Input: part model. Units: mm. Frame: model coordinates. A direction names the side the tool comes from. Give positions to 0.01 mm unless a question says otherwise; leave off trailing zeros. Loops run counter-clockwise (first coordinate to the right, second up) from the corner with the lowest first, then second, coordinate; pieces in that order, holes last. Notation, with made-up numbers: M 30.25,12.5 L 49.25,12.5 A24 ccw 49.25,42.5 Z; hole C 78,21.5 d4. An arc over 180 degrees is marked long. One line per item, written item: value. Start each with the question number.
(1) Pull-direction query (Y, two-part tool) for faces 1 (the flat face through (212, 12, 320.3)), 2 (the flat face through (212, -2, 310.475)), 3 (the flat face through (212.02, -3.6, 308.96)), 4 (the flat face through (218, 0, 301)); classes: released by +Y, released by -Y, zero draft, split by the parting line, or undercut.
(2) Pin query (flat end, axial travel): P1, Ø0.5, axis at x = 211, y = 18.5, coming from the -Z side; P2, Ø3, axis at x = 226.5, z = 302.5, coming from the +Y side; P3, Ø0.7, axis at y = 11.5, z = 319.5, coming from the -X side; P4, Ø8, axis at x = 240.5, z = 316.5, coming from the -Y side. Return the tip coordinate at first contact, or that it passes through.
(3) Section B-B on y = 20. Output: boundary loops of the cut face in (x, z).
(4) Section D-D on z = 313. Output: boundary loops of the cut face in (x, y), plus the area to 3 significant figures.
(5) Access query for faces 5 (the flat face through (212.02, 10.54, 308.96)), 6 (the flat face through (212, -5, 307.4)), 7 (the flat face through (212, 30.5, 310.475)), 8 (the flat face through (224.8, -0.7, 300.8)). Directions: +Z, -Z, +X, -X, +Y, -Y. A direction counts if a zero-diameter tool reaches every point of the face in a straight line with its end or side. Return the directions, or none.
(6) Section A-A on z = 303. Output: boundary loops of the cut face in (x, y).
(7) Ray query, line 1 along X through (y, z) = (25.5, 316); line 2 along Y through (x, z) = (218, 287.5); line 3 along X through (y, z) = (-0.5, 312). Return the intervals inside material, ascending. Write a range as from..to.
(8) Section C-C on x = 216.5. Output: boundary loops of the cut face in (y, z).
```python
from build123d import *

# Parameters (mm, degrees)
BOSS_EXTRUDE1_DEPTH = 4.7
SKETCH2_W           = 2.4
SKETCH2_H           = 37
BOSS_EXTRUDE2_DEPTH = 2
SKETCH3_W           = 7.4
SKETCH3_H           = 6
BOSS_EXTRUDE3_DEPTH = 0.8
SKETCH4_W           = 31
SKETCH4_H           = 6
BOSS_EXTRUDE4_DEPTH = 30
CUT_EXTRUDE4_DEPTH  = 4.7
SKETCH9_W           = 3
SKETCH9_H           = 6
BOSS_EXTRUDE6_DEPTH = 30
CUT_EXTRUDE5_DEPTH  = 405.447882922
CUT_EXTRUDE6_DEPTH  = 405.447882922
CUT_EXTRUDE7_DEPTH  = 6.5


with BuildPart() as part:
    # Sketch1 → Boss-Extrude1 (new body)
    with BuildSketch(Plane(origin=(209.7, 0, 0), x_dir=(0, 0, -1), z_dir=(1, 0, 0))):
        Polygon((-318, -6), (-318, 31), (-310.475, 31), (-310.475, 30.0599), (-307.4, 28.9407), (-307.4, 27.608), (-310.475, 26.4888), (-310.475, 25.3475), (-307.4, 24.2283), (-307.4, 22.8956), (-310.475, 21.7764), (-310.475, 20.6351), (-307.4, 19.5159), (-307.4, 18.1832), (-310.475, 17.064), (-310.475, 15.9227), (-307.4, 14.8035), (-307.4, 13.4708), (-310.475, 12.3516), (-310.475, 11.2103), (-307.4, 10.0911), (-307.4, 8.7584), (-310.475, 7.6392), (-310.475, 6.4979), (-307.4, 5.3787), (-307.4, 4.0461), (-310.475, 2.9268), (-310.475, 1.7855), (-307.4, 0.6663), (-307.4, -0.6663), (-310.475, -1.7855), (-310.475, -2.9268), (-307.4, -4.0461), (-307.4, -5.3787), (-309.1069, -6), align=None)
    extrude(amount=BOSS_EXTRUDE1_DEPTH)

    # Sketch2 → Boss-Extrude2 (add)
    with BuildSketch(Plane(origin=(211, 0, 0), x_dir=(0, 0, -1), z_dir=(1, 0, 0))):
        with Locations((-319.1, 12.5)):
            Rectangle(SKETCH2_W, SKETCH2_H)
    extrude(amount=BOSS_EXTRUDE2_DEPTH)

    # Sketch3 → Boss-Extrude3 (add)
    with BuildSketch(Plane(origin=(214.4, 0, 0), x_dir=(0, 0, -1), z_dir=(1, 0, 0))):
        with Locations((-314.3, -3)):
            Rectangle(SKETCH3_W, SKETCH3_H)
    extrude(amount=BOSS_EXTRUDE3_DEPTH)

    # Sketch4 → Boss-Extrude4 (add)
    with BuildSketch(Plane(origin=(215, 0, 0), x_dir=(0, 0, -1), z_dir=(1, 0, 0))):
        with Locations((-302.5, -3)):
            Rectangle(SKETCH4_W, SKETCH4_H)
    extrude(amount=BOSS_EXTRUDE4_DEPTH)

    # Sketch8 → Cut-Extrude4 (cut, symmetric)
    with BuildSketch(Plane(origin=(209.7, 0, 0), x_dir=(0, 0, -1), z_dir=(1, 0, 0))):
        Polygon((-307, -4.1716), (-310.475, -2.907), (-310.475, -3.047), (-307, -4.3116), align=None)
        Polygon((-307, -5.2532), (-310.475, -6.5178), (-310.475, -6.3778), (-307, -5.1132), align=None)
        Polygon((-307, 0.5408), (-310.475, 1.8054), (-310.475, 1.6654), (-307, 0.4008), align=None)
        Polygon((-307, -0.5408), (-310.475, -1.8054), (-310.475, -1.6654), (-307, -0.4008), align=None)
        Polygon((-307, 5.2532), (-310.475, 6.5178), (-310.475, 6.3778), (-307, 5.1132), align=None)
        Polygon((-307, 4.1716), (-310.475, 2.907), (-310.475, 3.047), (-307, 4.3116), align=None)
        Polygon((-307, 9.9656), (-310.475, 11.2302), (-310.475, 11.0902), (-307, 9.8256), align=None)
        Polygon((-307, 8.884), (-310.475, 7.6194), (-310.475, 7.7594), (-307, 9.024), align=None)
        Polygon((-307, 14.678), (-310.475, 15.9426), (-310.475, 15.8026), (-307, 14.538), align=None)
        Polygon((-307, 13.5964), (-310.475, 12.3318), (-310.475, 12.4718), (-307, 13.7364), align=None)
        Polygon((-307, 19.3904), (-310.475, 20.655), (-310.475, 20.515), (-307, 19.2504), align=None)
        Polygon((-307, 18.3088), (-310.475, 17.0442), (-310.475, 17.1842), (-307, 18.4488), align=None)
        Polygon((-307, 24.1027), (-310.475, 25.3673), (-310.475, 25.2274), (-307, 23.9628), align=None)
        Polygon((-307, 23.0211), (-310.475, 21.7565), (-310.475, 21.8965), (-307, 23.1611), align=None)
        Polygon((-307, 28.8151), (-310.475, 30.0797), (-310.475, 29.9397), (-307, 28.6751), align=None)
        Polygon((-307, 27.7335), (-310.475, 26.4689), (-310.475, 26.6089), (-307, 27.8735), align=None)
    extrude(amount=CUT_EXTRUDE4_DEPTH, both=True, mode=Mode.SUBTRACT)

    # Sketch9 → Boss-Extrude6 (add)
    with BuildSketch(Plane(origin=(215, 0, 0), x_dir=(0, 0, -1), z_dir=(1, 0, 0))):
        with Locations((-285.5, -3)):
            Rectangle(SKETCH9_W, SKETCH9_H)
    extrude(amount=BOSS_EXTRUDE6_DEPTH)

    # Sketch10 → Cut-Extrude5 (cut, through all)
    with BuildSketch(Plane.XY):
        Polygon((227.5, -6.5), (246.5, -2.7), (246.5, -6.5), align=None)
    extrude(amount=CUT_EXTRUDE5_DEPTH, mode=Mode.SUBTRACT)

    # Sketch11 → Cut-Extrude6 (cut, through all)
    with BuildSketch(Plane.XY):
        Polygon((222, 0.5), (226, 0.5), (224, -1.5), align=None)
    extrude(amount=CUT_EXTRUDE6_DEPTH, mode=Mode.SUBTRACT)

    # Sketch12 → Cut-Extrude7 (cut, symmetric)
    with BuildSketch(Plane(origin=(0, 0, 0), x_dir=(1, 0, 0), z_dir=(0, 1, 0))):
        Polygon((228.125, -319.1875), (246.5, -307.55), (246.5, -319.1875), align=None)
        Polygon((228.125, -282.8125), (246.5, -294.45), (246.5, -282.8125), align=None)
    extrude(amount=CUT_EXTRUDE7_DEPTH, both=True, mode=Mode.SUBTRACT)


solid = part.part
```
Output values:
1. face 1: zero draft
1. face 2: undercut
1. face 3: undercut
1. face 4: released by +Y
2. P1: stops at z = 307.4
2. P2: stops at y = 0
2. P3: stops at x = 211
2. P4: passes through
3. outline: M 209.7,309.06 L 214.4,309.06 L 214.4,318 L 213,318 L 213,320.3 L 211,320.3 L 211,318 L 209.7,318 Z
4. outline: M 209.7,-6 L 230,-6 L 237.89,-4.42 L 237.89,0 L 225.5,0 L 224,-1.5 L 222.5,0 L 214.4,0 L 214.4,31 L 209.7,31 Z
4. area: 306 mm²
5. face 5: -Z, +X, -X
5. face 6: -Z, -X, +Y, -Y
5. face 7: -Z, +X, -X, +Y
5. face 8: +Z, -Z, +Y
6. outline: M 215,-6 L 230,-6 L 245,-3 L 245,0 L 225.5,0 L 224,-1.5 L 222.5,0 L 215,0 Z
7. line 1: x = 209.7..214.4
7. line 2: y = -6..0
7. line 3: x = 209.7..223, 225..239.47
8. outline: M -6,284 L 0,284 L 0,318 L -6,318 Z
